Check sheet for the drawn part. Datum: minimum x, y, z corner. Units: mm. A direction names the side the tool comes from. Coordinates: 2 decimals unless noted, no trailing zeros. Write each loop counter-clockwise with the first axis right and the second up, starting at its lowest first coordinate (ties: lowest second). Pieces come first, ordered by that corner, then holes. Notation, with made-up numbers: (14, 47) -> (39, 47) arc R23 cw to (39, 56) -> close; hole circle Ø5 at (-19.5, -18.75). An arc over 180 degrees is marked (long way). Answer in a Markdown table with one row per item.
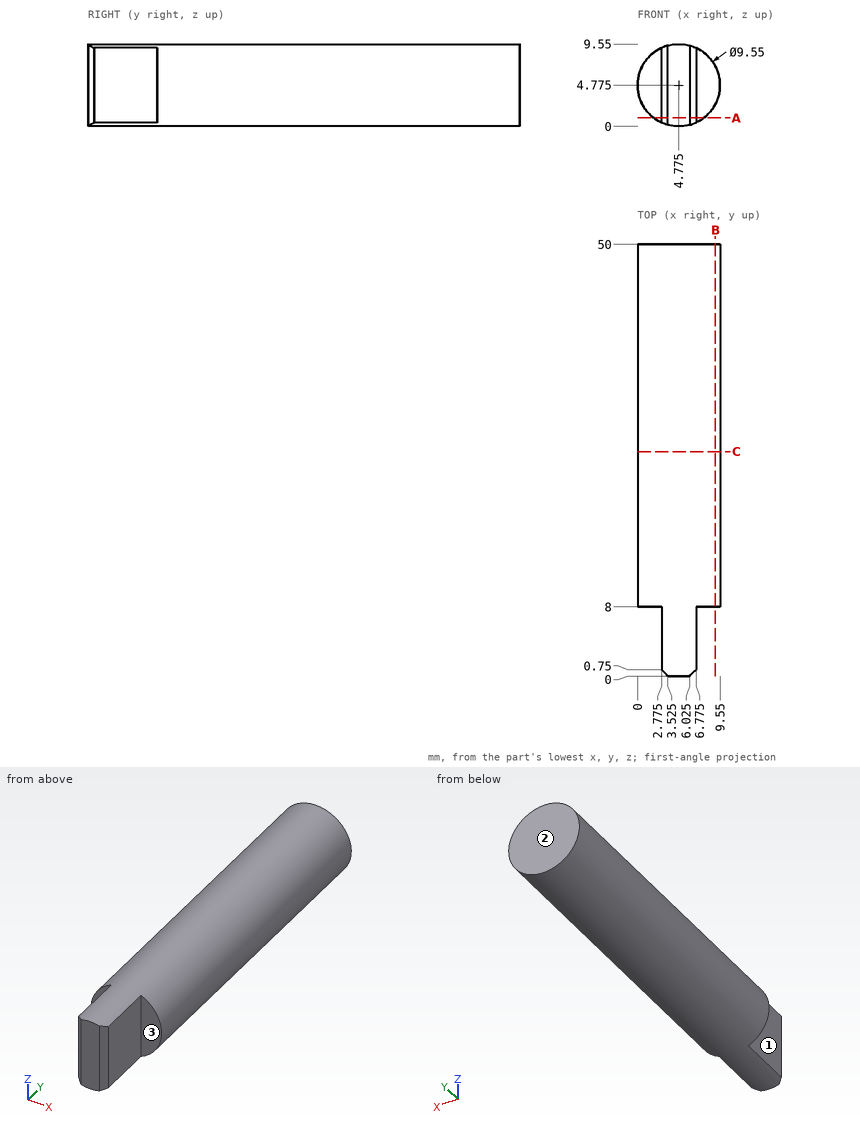
1. Go/stop test with flat-tipped pins: pin 1 (3.5 mm diameter, centred on y = 3.5, z = 6, fed in from +X) (3 decimals); pin 2 (2 mm diameter, centred on x = 8, z = 5.5, fed in from -Y); pin 3 (3 mm diameter, centred on x = 3, y = 13, fed in from -Z). Record where each tip stops, or that it passes through.
Findings below:
| item | result |
|---|---|
| pin 1 | stops at x = 6.775 |
| pin 2 | stops at y = 8 |
| pin 3 | stops at z = 0.01 |
2. Sectioned sample at A-A, the plane z = 1. Record the cut outline in (x, y) (3 decimals).
Findings below:
| item | result |
|---|---|
| outline | (1.851, 8) -> (2.775, 8) -> (2.775, 0.75) -> (3.525, 0) -> (6.025, 0) -> (6.775, 0.75) -> (6.775, 8) -> (7.699, 8) -> (7.699, 50) -> (1.851, 50) -> close |
3. Sectioned sample at B-B, the plane x = 9. Record the cut outline in (y, z).
Findings below:
| item | result |
|---|---|
| outline | (8, 2.55) -> (50, 2.55) -> (50, 7) -> (8, 7) -> close |
4. Access from +Z, -Z, +X, -X, +Y, -Y to the whole of each face (thin tool, end or side, straight path). Record for the marked faces 1, 2 and 3.
Findings below:
| item | result |
|---|---|
| face 1 | +Z, -Z, -X, -Y |
| face 2 | +Z, -Z, +X, -X, +Y |
| face 3 | +Z, -Z, +X, -Y |
5. Sectioned sample at C-C, the plane y = 26. Record the cut outline in (x, z) (3 decimals).
Findings below:
| item | result |
|---|---|
| outline | circle Ø9.55 at (4.775, 4.775) |
6. Material ranges on probe 1 along X at (y, z) = (3.5, 7.25) (3 decimals); probe 2 along X at (y, z) = (13, 3.5), recorded low to high. Write a range as from..to.
Findings below:
| item | result |
|---|---|
| probe 1 | x = 2.775..6.775 |
| probe 2 | x = 0.17..9.38 |
